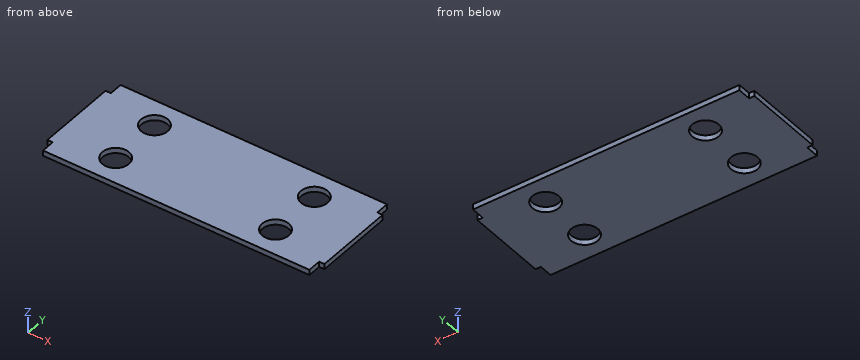
```python
from build123d import *

# Parameters (mm, degrees)
SKETCH_1_W          = 2
SKETCH_1_H          = 30
SKETCH_1_W_2        = 100
SKETCH_1_H_2        = 40
EXTRUDE_1_DEPTH     = 2
SKETCH_2_R          = 5
CUT_EXTRUDE_1_DEPTH = 110.581020254


with BuildPart() as part:
    # 草图1 → 凸台-拉伸1 (new body)
    with BuildSketch(Plane.XY):
        with Locations((-1, 20)):
            Rectangle(SKETCH_1_W, SKETCH_1_H)
        with Locations((50, 20)):
            Rectangle(SKETCH_1_W_2, SKETCH_1_H_2)
        with Locations((101, 20)):
            Rectangle(SKETCH_1_W, SKETCH_1_H)
    extrude(amount=EXTRUDE_1_DEPTH)

    # 草图2 → 切除-拉伸1 (cut, through all)
    with BuildSketch(Plane.XY):
        with Locations((20, 30)):
            Circle(SKETCH_2_R)
        with Locations((80, 30)):
            Circle(SKETCH_2_R)
        with Locations((80, 10)):
            Circle(SKETCH_2_R)
        with Locations((20, 10)):
            Circle(SKETCH_2_R)
    extrude(amount=CUT_EXTRUDE_1_DEPTH, mode=Mode.SUBTRACT)


solid = part.part
```
Work out the finished part from the listing and answer in its coordinate system (mm). Give positions to 0.01 mm unless a question says otherwise; leave off trailing zeros. Order: outer loops, then holes, each group sorted by start corner. A loop starts at its lowest first (then second) coordinate and runs counter-clockwise, first axis right, second up. Notation, with made-up numbers: (2.25, 76.5) -> (44.25, 76.5) arc R30 cw to (44.25, 108.5) -> close; hole circle Ø4 at (75.25, 8). An arc over 180 degrees is marked (long way). Answer as CSV lines item,"result". Start each with the question number.
(1) Section B-B, the plane x = 80 is taken. Write down the section's boundary in (y, z).
(2) Section A-A, the plane y = 30 is taken. Write down the section's boundary in (x, z), plus the area to 3 significant figures.
(3) Section D-D, the plane y = 36 is taken. Write down the section's boundary in (x, z).
(4) Section C-C, the plane z = 1.1 is taken. Write down the section's boundary in (x, y).
(5) Each of these flat-tipped pins is pushed along its axis until it touches: pin 1 Ø0.6 at (x, z) = (-1.5, 1.5) entering from +Y; pin 2 Ø1 at (y, z) = (3.5, 1) entering from +X; pin 3 Ø0.6 at (y, z) = (2, 1) entering from -X. Where does it stop, or does it pass through?
(6) Consider line 1 along Y through (x, z) = (20, 0.65); line 2 along X through (y, z) = (10, 1.35); line 3 along X through (y, z) = (7, 1.55). Determine where each line is inside the solid, lowest interval first.
Entries:
1,outline,"(0, 0) -> (5, 0) -> (5, 2) -> (0, 2) -> close; (15, 0) -> (25, 0) -> (25, 2) -> (15, 2) -> close; (35, 0) -> (40, 0) -> (40, 2) -> (35, 2) -> close"
2,outline,"(-2, 0) -> (15, 0) -> (15, 2) -> (-2, 2) -> close; (25, 0) -> (75, 0) -> (75, 2) -> (25, 2) -> close; (85, 0) -> (102, 0) -> (102, 2) -> (85, 2) -> close"
2,area,"168 mm²"
3,outline,"(0, 0) -> (100, 0) -> (100, 2) -> (0, 2) -> close"
4,outline,"(-2, 5) -> (0, 5) -> (0, 0) -> (100, 0) -> (100, 5) -> (102, 5) -> (102, 35) -> (100, 35) -> (100, 40) -> (0, 40) -> (0, 35) -> (-2, 35) -> close; hole circle Ø10 at (20, 10); hole circle Ø10 at (20, 30); hole circle Ø10 at (80, 10); hole circle Ø10 at (80, 30)"
5,pin 1,"y = 35"
5,pin 2,"x = 100"
5,pin 3,"x = 0"
6,line 1,"0 to 5, 15 to 25, 35 to 40"
6,line 2,"-2 to 15, 25 to 75, 85 to 102"
6,line 3,"-2 to 16, 24 to 76, 84 to 102"
